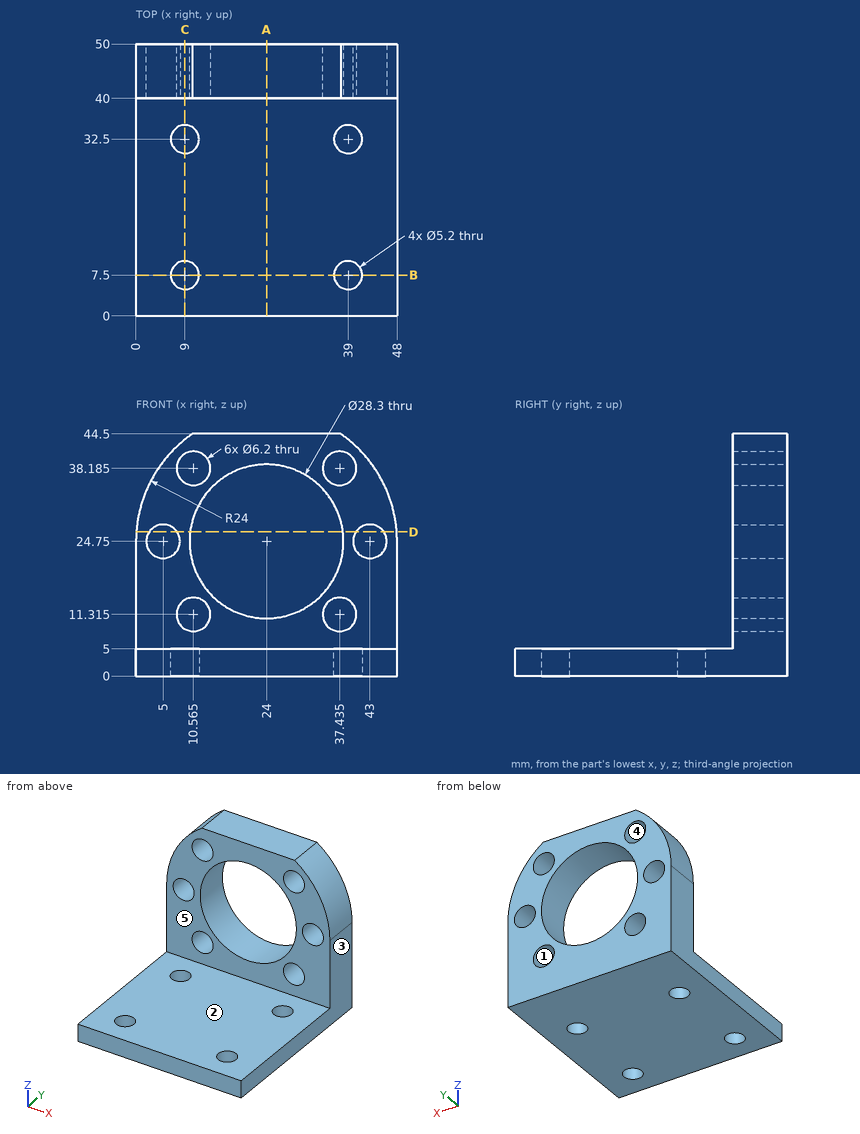
Drawing for the job (mm, zero at the part's lowest x, y, z). A direction names the side the tool comes from. Round coordinates to 2 decimals unless told otherwise and drop trailing zeros. Loops run counter-clockwise (first coordinate to the right, second up) from the corner with the lowest first, then second, coordinate; pieces in that order, holes last. Notation, with made-up numbers: (88.5, 58.25) -> (119.5, 58.25) arc R15 cw to (119.5, 71.25) -> close; hole circle Ø5 at (10, 15). An arc over 180 degrees is marked (long way). Answer in a Markdown table with one row per item.
Item 1: Saw through at C-C (x = 9). Write the cut outline in (y, z) (3 decimals).
Answers below:
| item | result |
|---|---|
| outline | (0, 0) -> (4.9, 0) -> (4.9, 5) -> (0, 5) -> close; (10.1, 0) -> (29.9, 0) -> (29.9, 5) -> (10.1, 5) -> close; (35.1, 0) -> (50, 0) -> (50, 8.639) -> (40, 8.639) -> (40, 5) -> (35.1, 5) -> close; (40, 13.991) -> (50, 13.991) -> (50, 35.509) -> (40, 35.509) -> close; (40, 40.861) -> (50, 40.861) -> (50, 43.485) -> (40, 43.485) -> close |
Item 2: Saw through at A-A (x = 24). Write the cut outline in (y, z).
Answers below:
| item | result |
|---|---|
| outline | (0, 0) -> (50, 0) -> (50, 10.6) -> (40, 10.6) -> (40, 5) -> (0, 5) -> close; (40, 38.9) -> (50, 38.9) -> (50, 44.5) -> (40, 44.5) -> close |
Item 3: Drill centre lines: L1, parallel to X at y = 7, z = 2; L2, parallel to Z at x = 39, y = 48.5 (3 decimals); L3, parallel to Z at x = 24, y = 43.5. Where is each one in solid material? Low to high. Write a range as [from, to].
Answers below:
| item | result |
|---|---|
| L1 | x = [0, 6.45], [11.55, 36.45], [41.55, 48] |
| L2 | z = [0, 8.639], [13.991, 35.509], [40.861, 43.485] |
| L3 | z = [0, 10.6], [38.9, 44.5] |
Item 4: Saw through at D-D (z = 26.5). Write the cut outline in (x, y).
Answers below:
| item | result |
|---|---|
| outline | (0.06, 40) -> (2.44, 40) -> (2.44, 50) -> (0.06, 50) -> close; (7.56, 40) -> (9.96, 40) -> (9.96, 50) -> (7.56, 50) -> close; (38.04, 40) -> (40.44, 40) -> (40.44, 50) -> (38.04, 50) -> close; (45.56, 40) -> (47.94, 40) -> (47.94, 50) -> (45.56, 50) -> close |
Item 5: Saw through at B-B (y = 7.5). Write the cut outline in (x, z).
Answers below:
| item | result |
|---|---|
| outline | (0, 0) -> (6.4, 0) -> (6.4, 5) -> (0, 5) -> close; (11.6, 0) -> (36.4, 0) -> (36.4, 5) -> (11.6, 5) -> close; (41.6, 0) -> (48, 0) -> (48, 5) -> (41.6, 5) -> close |
Item 6: Which spindle directions (+Z, -Z, +X, -X, +Y, -Y) get a long thin tool onto all of the face, cutting with end or side? Do the marked faces 4 and 5. Say none if no direction does.
Answers below:
| item | result |
|---|---|
| face 4 | +Y, -Y |
| face 5 | +Z, +X, -X, -Y |
Item 7: Pin check, flat tips, straight feed: pin 1 (8 mm diameter, centred on x = 37.44, z = 38.19, fed in from -Y); pin 2 (3 mm diameter, centred on x = 39, y = 32.5, fed in from -Z); pin 3 (12 mm diameter, centred on x = 15, y = 31.5, fed in from +Z). Stop position of each tip, or through.
Answers below:
| item | result |
|---|---|
| pin 1 | stops at y = 40 |
| pin 2 | passes through |
| pin 3 | stops at z = 5 |
Item 8: Mould opens along X. For the marked faces 1, 2 and 3 say: +X half, -X half, draft (parallel to the pull), parting line (faces both ways), or undercut.
Answers below:
| item | result |
|---|---|
| face 1 | undercut |
| face 2 | draft |
| face 3 | +X half |
